Job drawing, mm, ordinate dimensions from the low corner. One solid piece. Round coordinates to 2 decimals unless told otherwise and drop trailing zeros. Loops run counter-clockwise (first coordinate to the right, second up) from the corner with the lowest first, then second, coordinate; pieces in that order, holes last.
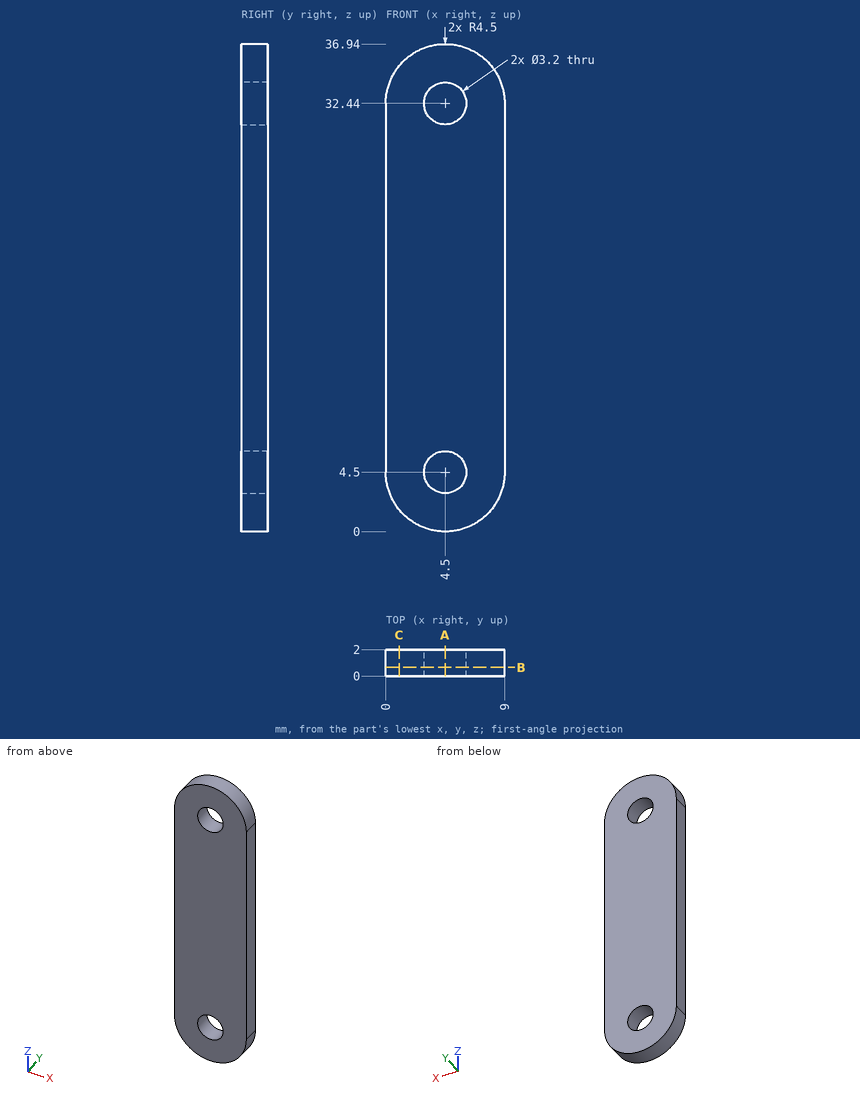
(1) Slice it at B-B on y = 0.65. List the corners of the cut face in (x, z), plus the area to 3 significant figures.
Responses:
outline: (0, 4.5) arc R4.5 ccw to (9, 4.5) - (9, 32.44) arc R4.5 ccw to (0, 32.44) - close; hole circle Ø3.2 at (4.5, 4.5); hole circle Ø3.2 at (4.5, 32.44)
area: 299 mm2
(2) Slice it at A-A on x = 4.5. List the corners of the cut face in (y, z).
Responses:
outline: (0, 0) - (2, 0) - (2, 2.9) - (0, 2.9) - close; (0, 6.1) - (2, 6.1) - (2, 30.84) - (0, 30.84) - close; (0, 34.04) - (2, 34.04) - (2, 36.94) - (0, 36.94) - close
(3) Slice it at C-C on x = 1. List the corners of the cut face in (y, z).
Responses:
outline: (0, 1.67) - (2, 1.67) - (2, 35.27) - (0, 35.27) - close
(4) Probe line 1 (X direction, y = 1.1, z = 32.44); line 2 (Z direction, x = 5.5, y = 0.5); line 3 (Z direction, x = 4, y = 1.75). List the from-to ranges inside material, lowest first.
Responses:
line 1: x = 0 to 2.9, 6.1 to 9
line 2: z = 0.11 to 3.25, 5.75 to 31.19, 33.69 to 36.83
line 3: z = 0.03 to 2.98, 6.02 to 30.92, 33.96 to 36.91
